from build123d import *

# Parameters (mm, degrees)
SALIENTE_EXTRUIR1_DEPTH = 314
CORTAR_EXTRUIR1_DEPTH   = 2


with BuildPart() as part:
    # Croquis2 → Saliente-Extruir1 (new body)
    with BuildSketch(Plane(origin=(0, 0, 0), x_dir=(0, 0, -1), z_dir=(1, 0, 0))):
        with BuildLine():
            Line((-38.572123539, -20.408891327), (-38.572123539, 101.591108673))
            ThreePointArc((-38.572123539, 101.591108673), (-23.927462599, 136.946447732), (11.427876461, 151.591108673))
            Line((11.427876461, 151.591108673), (131.427876461, 151.591108673))
            Line((131.427876461, 151.591108673), (131.427876461, 147.591108673))
            Line((131.427876461, 147.591108673), (15.427876461, 147.591108673))
            ThreePointArc((15.427876461, 147.591108673), (-19.927462599, 132.946447732), (-34.572123539, 97.591108673))
            Line((-34.572123539, 97.591108673), (-34.572123539, -20.408891327))
            Line((-34.572123539, -20.408891327), (-38.572123539, -20.408891327))
        make_face()
    extrude(amount=-SALIENTE_EXTRUIR1_DEPTH)

    # Croquis3 → Cortar-Extruir1 (cut)
    with BuildSketch(Plane(origin=(0, 0, 34.572123539), x_dir=(-1, 0, 0), z_dir=(0, 0, -1))):
        Polygon((2, 97.591108673), (2, -18.408891327), (312, -18.408891327), (312, 97.591108673), (308, 97.591108673), (308, -14.408891327), (6, -14.408891327), (6, 97.591108673), align=None)
    extrude(amount=-CORTAR_EXTRUIR1_DEPTH, mode=Mode.SUBTRACT)


solid = part.part
Source: CAD feature listing. Evaluate the final solid. Frame: model axes, mm. A direction names the side the tool comes from. Coordinates: 2 decimals unless noted, no trailing zeros. Loops run counter-clockwise (first coordinate to the right, second up) from the corner with the lowest first, then second, coordinate; pieces in that order, holes last. Notation, with made-up numbers: (-29.75, 39.5) - (-8.75, 39.5) arc R17 ccw to (-8.75, 46.5) - close; hole circle Ø5 at (7.25, 12.5). An arc over 180 degrees is marked (long way). One line per item, written item: value. Start each with the question number.
1. Section C-C (z = -105.5). Return the cut outline in (x, y).
2. Ray query, L1, parallel to Z at x = -128.5, y = 42; L2, parallel to Y at x = -191, z = -55; L3, parallel to Z at x = -198, y = 127. Return the intervals inside material, ascending.
3. Set-up query: faces 1 (the flat face through (-155, 42, 34.572)), 2 (the flat face through (-155, 151.591, -71)). Return all of +Z, -Z, +X, -X, +Y, -Y with unobstructed straight access to the full face (end or side cutting, diameter ignored); none if empty.
4. Section B-B (y = 73.5). Return the cut outline in (x, z).
5. Section A-A (x = -104.5). Return the cut outline in (y, z), and give its area (3 significant figures).
6. Mould query, pull axis X, two halves, no side actions, for faces 3 (the flat face through (0, 123, 29)), 4 (the flat face through (-156, -16, 36.572)), 5 (the flat face through (-314, 123, 29)), 6 (the flat face through (-155, 147.591, -74)). Classes: pulls with the +X half, pulls with the -X half, needs draft (parallel to the pull), parting line crosses it, or undercut.
7. Contact query for flat-ended pins moving along their axis: P1, Ø1.6, axis at x = -105, z = 35.5, coming from the +Y side; P2, Ø1, axis at y = 32.5, z = 35, coming from the +X side; P3, Ø8, axis at x = -185, y = 57.5, coming from the -Z side; P4, Ø6, axis at x = -243.5, z = -49.5, coming from the -Y side. Output: stop coordinate, or through.
8. Section D-D (z = 26). Return the cut outline in (x, y), and give its area (3 significant figures).
Verdict:
1. outline: (-314, 147.59) - (0, 147.59) - (0, 151.59) - (-314, 151.59) - close
2. L1: z = 34.57 to 38.57
2. L2: y = 147.59 to 151.59
2. L3: z = 25.01 to 31.63
3. face 1: -Z, +X, -X, -Y
3. face 2: +Z, -Z, +X, -X, +Y
4. outline: (-314, 34.57) - (-312, 34.57) - (-312, 36.57) - (-308, 36.57) - (-308, 34.57) - (-6, 34.57) - (-6, 36.57) - (-2, 36.57) - (-2, 34.57) - (0, 34.57) - (0, 38.57) - (-314, 38.57) - close
5. outline: (-20.41, 34.57) - (-18.41, 34.57) - (-18.41, 36.57) - (-14.41, 36.57) - (-14.41, 34.57) - (97.59, 34.57) arc R50 cw to (147.59, -15.43) - (147.59, -131.43) - (151.59, -131.43) - (151.59, -11.43) arc R50 ccw to (101.59, 38.57) - (-20.41, 38.57) - close
5. area: 1,340 mm2
6. face 3: pulls with the +X half
6. face 4: undercut
6. face 5: pulls with the -X half
6. face 6: needs draft
7. P1: stops at y = 120.88
7. P2: stops at x = 0
7. P3: stops at z = 34.57
7. P4: stops at y = 147.59
8. outline: (-314, 125.59) - (0, 125.59) - (0, 134.74) - (-314, 134.74) - close
8. area: 2,880 mm2
